Work out the finished part from the listing and answer in its coordinate system (mm). A direction names the side the tool comes from. Coordinates: 2 decimals unless noted, no trailing zeros. Order: outer loops, then holes, each group sorted by start corner. A loop starts at its lowest first (then second) coordinate and runs counter-clockwise, first axis right, second up.
```python
from build123d import *

# Parameters (mm, degrees)
BINDER_W          = 42.6
BINDER_H          = 40.6
PAD002_DEPTH      = 16.3
SKETCH_R          = 1.8
PAD_DEPTH         = 2
SKETCH003_W       = 13.1
SKETCH003_H       = 1114
PAD001_DEPTH      = 7.3
SKETCH004_W       = 15
SKETCH004_H       = 20
PAD003_DEPTH      = 8.3
PAD003_DEPTH_BACK = 1


with BuildPart() as part:
    # Binder → Pad002 (new body)
    with BuildSketch(Plane(origin=(11.3, 21.3, 0), x_dir=(0, 1, 0), z_dir=(0, 0, 1))):
        Rectangle(BINDER_W, BINDER_H)
    extrude(amount=PAD002_DEPTH)

    # Sketch → Pad (join)
    with BuildSketch(Plane(origin=(11.1, 0, 0), x_dir=(-1, 0, 0), z_dir=(0, 0, 1))):
        with BuildLine():
            ThreePointArc((4.5, 4), (0, 8.5), (-4.5, 4))
            Line((-4.5, 4), (-4.5, 0))
            Line((-4.5, 0), (4.5, 0))
            Line((4.5, 0), (4.5, 4))
        make_face()
        with Locations((0, 4)):
            Circle(SKETCH_R, mode=Mode.SUBTRACT)
    extrude(amount=PAD_DEPTH)

    # Sketch003 → Pad001 (join)
    with BuildSketch(Plane.XY):
        with Locations((0, -557)):
            Rectangle(SKETCH003_W, SKETCH003_H)
    extrude(amount=PAD001_DEPTH)

    # Sketch004 → Pad003 (join, two sides)
    with BuildSketch(Plane.XY) as pad003_sk:
        with Locations((0, -1124)):
            Rectangle(SKETCH004_W, SKETCH004_H)
    extrude(amount=PAD003_DEPTH)
    extrude(pad003_sk.sketch, amount=-PAD003_DEPTH_BACK)


solid = part.part
```
1. The part is cut by section B-B (z = 11.5). Determine the outline of the cut face in (x, y), plus the area to 3 significant figures.
2. Consider probe 1 along Y at (x, z) = (11.1, 0.85); probe 2 along Y at (x, z) = (22, 2.5); probe 3 along X at (y, z) = (-618, 2). Determine where each line is inside the solid, lowest interval first.
3. Flat-ended cylindrical pins translate along their axes: pin 1 (6 mm diameter, centred on x = 18, z = 10.5, fed in from -Y); pin 2 (0.6 mm diameter, centred on y = -3, z = 1.5, fed in from +X); pin 3 (2.5 mm diameter, centred on x = 12.5, y = -4, fed in from +Z). Find the tip coordinate at first contact, or state that the pin passes through.
4. For faces 1 (the flat face through (-1, -490, 0)), 2 (the flat face through (11, 21, 16.3)), determine the directions among +Z, -Z, +X, -X, +Y, -Y from which every point of the face is accessible in a straight line to the end or side of a thin tool.
5. The part is cut by section A-A (y = -235). Determine the outline of the cut face in (x, z).
Worked out:
1. outline: (-9, 0) - (31.6, 0) - (31.6, 42.6) - (-9, 42.6) - close
1. area: 1,730 mm2
2. probe 1: y = -8.5 to -5.8, -2.2 to 42.6
2. probe 2: y = 0 to 42.6
2. probe 3: x = -6.55 to 6.55
3. pin 1: stops at y = 0
3. pin 2: stops at x = 15.6
3. pin 3: stops at z = 2
4. face 1: -Z, +X, -X, +Y
4. face 2: +Z, +X, -X, +Y, -Y
5. outline: (-6.55, 0) - (6.55, 0) - (6.55, 7.3) - (-6.55, 7.3) - close
